Autodesk Inventor part; units mm, degrees
ref_plane "Work Plane1" through (0, 0, -15) normal (0, 0, 1) x (1, 0, 0)
ref_plane "YZ Plane" through (0, 0, 0) normal (1, 0, 0) x (0, 1, 0)
ref_plane "XZ Plane" through (0, 0, 0) normal (0, 1, 0) x (-1, 0, 0)
sketch "Sketch1" plane through (0, 0, 0) normal (0, 0, 1) x (1, 0, 0)
  line L0 (0, 0) -> (25, 0)
  line L1 (25, 0) -> (25, 40)
  line L2 (25, 40) -> (0, 40)
  line L3 (0, 40) -> (0, 0)
  dimension "d1" = 25
  dimension "d2" = 40
  dimension "d3" = 25
extrude "Extrusion1" add sketch "Sketch1" against normal blind 30
sketch "Sketch2" plane through (25, 0, 0) normal (1, 0, 0) x (0, 0, -1)
  line L0 (0, 0) -> (30, 0)
  circle A0 centre (15, 6.56) radius 2.46
extrude "Extrusion2" cut sketch "Sketch2" against normal blind 30
sketch "Sketch3" plane through (0, 0, 0) normal (-1, 0, 0) x (0, 0, 1)
  line L0 (0, 0) -> (-30, 0)
  line L1 (-25.05, 0) -> (-4.95, 0)
  line L2 (-4.95, 0) -> (-4.95, 33.12)
  line L3 (-4.95, 33.12) -> (-25.05, 33.12)
  line L4 (-25.05, 33.12) -> (-25.05, 0)
  dimension "d11" = 20.1
extrude "Extrusion3" cut sketch "Sketch3" against normal blind 20
sketch "Sketch4" plane through (0, 0, 0) normal (0, -1, 0) x (1, 0, 0)
  line L0 (20, -4.95) -> (20, -25.05)
  line L1 (20, -15) -> (25, -15)
  line L2 (25, 0) -> (25, -30)
  line L3 (20, -8.025) -> (25, -8.025)
  line L4 (25, -8.025) -> (25, -21.975)
  line L5 (25, -21.975) -> (20, -21.975)
  line L6 (20, -21.975) -> (20, -8.025)
  line L7 (20, -8.025) -> (25, -21.975) construction
  line L8 (25, -8.025) -> (20, -21.975) construction
  line L9 (25, -12.54) -> (25, -17.46)
  point P0 (0, 0)
  point P1 (22.5, -15)
  dimension "d14" = 13.95
extrude "Extrusion4" add sketch "Sketch4" along normal blind 15
sketch "Sketch5" plane through (20, 0, 0) normal (-1, 0, 0) x (0, 0, 1)
  circle A0 centre (-15, 6.56) radius 2.46
  circle A1 centre (-15, 6.56) radius 4.7025
  circle A2 centre (-15, 6.56) radius 2.46
  circle A3 centre (-15, 6.56) radius 2.46
  point P0 (0, 0)
  dimension "d17" = 9.405
extrude "Extrusion5" cut sketch "Sketch5" against normal blind 2.1
sketch "Sketch6" plane through (25, 0, 0) normal (1, 0, 0) x (0, 0, -1)
  circle A0 centre (15, 6.56) radius 4.7025
  line L0 (15, 6.56) -> (15, 23.56)
  circle A1 centre (15, 23.56) radius 2.46
  point P0 (0, 0)
  dimension "d20" = 17
  dimension "d21" = 4.92
extrude "Extrusion6" cut sketch "Sketch6" against normal blind 10 contours A1
sketch "Sketch7" plane through (20, 0, 0) normal (-1, 0, 0) x (0, 0, 1)
  circle A0 centre (-15, 23.56) radius 2.46
  circle A1 centre (-15, 23.56) radius 4.7025
  point P0 (0, 0)
  dimension "d24" = 9.405
extrude "Extrusion7" cut sketch "Sketch7" against normal blind 2.1
sketch "Sketch9" plane through (25, 0, 0) normal (1, 0, 0) x (0, 0, -1)
  circle A0 centre (15, 6.56) radius 2.46
  circle A1 centre (15, 6.56) radius 2.46
  circle A2 centre (15, 23.56) radius 2.46
  circle A3 centre (15, 23.56) radius 2.46
  line L0 (30, 40) -> (30, 0)
  line L1 (30, 0) -> (30, 40)
  line L2 (30, 40) -> (0, 40)
  line L3 (0, 40) -> (0, 0)
  line L4 (0, 0) -> (8.025, 0)
  line L5 (21.975, 0) -> (21.975, -15)
  line L6 (21.975, -15) -> (8.025, -15)
  line L7 (8.025, -15) -> (8.025, 0)
  line L8 (0, 0) -> (8.025, 0)
  line L9 (21.975, 0) -> (30, 0)
extrude "Extrusion8" add sketch "Sketch9" along normal blind 5
sketch "Sketch10" plane through (0, 40, 0) normal (0, 1, 0) x (1, 0, 0)
  line L0 (0, 30) -> (30, 30)
  line L1 (30, 0) -> (0, 0)
  line L2 (0, 30) -> (30, 30)
  line L3 (30, 30) -> (30, 0)
  line L4 (30, 0) -> (0, 0)
  line L5 (0, 0) -> (0, 30)
extrude "Extrusion9" add sketch "Sketch10" along normal blind 30
sketch "Sketch12" plane through (30, 0, 0) normal (1, 0, 0) x (0, 0, -1)
  circle A0 centre (15, 6.56) radius 2.46
  line L0 (15, 6.56) -> (15, 15.06)
  circle A1 centre (15, 15.06) radius 2.525
  point P0 (0, 0)
  dimension "d31" = 8.5
  dimension "d33" = 5.05
extrude "Extrusion10" cut sketch "Sketch12" against normal blind 30 contours A1
sketch "Sketch14" plane through (0, 0, 0) normal (0, 0, 1) x (1, 0, 0)
  line L0 (30, 70) -> (0, 70)
  line L1 (0, 70) -> (0, 85)
  line L2 (-15, 100) -> (-23, 100)
  line L3 (30, 0) -> (30, 70)
  line L4 (30, 118) -> (30, 70)
  arc A0 (0, 85) -> (-15, 100) centre (-15, 85) ccw
  line L5 (30, 105) -> (30, 100)
  line L6 (-18, 134) -> (-23, 136)
  line L7 (-18, 102) -> (-23, 100)
  line L8 (-18, 102) -> (-13, 118)
  line L9 (-13, 118) -> (-18, 134)
  line L10 (15, 136) -> (30, 118)
  line L11 (-23, 136) -> (15, 136)
  point P0 (0, 0)
  point P1 (0, 100)
  dimension "d47" = 30
  dimension "d54" = 15
extrude "Extrusion12" add sketch "Sketch14" against normal blind 30
sketch "Sketch15" plane through (0, 0, -25.05) normal (-1, 0, 0) x (0, 0, 1)
  line L0 (0, 33.12) -> (20.1, 33.12)
  line L1 (20.1, 33.12) -> (20.1, 0)
  line L2 (0, 33.12) -> (20.1, 33.12)
  line L3 (20.1, 33.12) -> (20.1, 31.1)
  line L4 (20.1, 31.1) -> (0, 31.1)
  line L5 (0, 31.1) -> (0, 33.12)
  point P0 (25.05, 0)
  dimension "d57" = 2.02
extrude "Extrusion13" add sketch "Sketch15" against normal blind 20
sketch "Sketch22" plane through (0, 0, 0) normal (0, 0, 1) x (1, 0, 0)
  line L0 (-15, 100) -> (-23, 100)
  line L1 (-15, 100) -> (-23, 100)
  line L2 (-23, 100) -> (-18, 102)
  line L3 (-23, 100) -> (-18, 102)
  line L4 (-18, 102) -> (-13, 118)
  line L5 (-18, 102) -> (-13, 118)
  line L6 (-13, 118) -> (-18, 134)
  line L7 (-13, 118) -> (-18, 134)
  line L8 (-18, 134) -> (-23, 136)
  line L9 (-18, 134) -> (-23, 136)
  line L10 (-23, 136) -> (15, 136)
  line L11 (-23, 136) -> (15, 136)
  line L12 (15, 136) -> (30, 118)
  line L13 (15, 136) -> (30, 118)
  line L14 (30, 118) -> (30, 78)
  line L15 (30, 0) -> (30, 118)
  line L16 (30, 78) -> (0, 78)
  arc A0 (0, 85) -> (-15, 100) centre (-15, 85) ccw
  line L17 (0, 78) -> (0, 85)
  arc A1 (0, 85) -> (-15, 100) centre (-15, 85) ccw
  point P0 (0, 0)
  dimension "d82" = 40
extrude "Extrusion14" add sketch "Sketch22" along normal blind 15
ref_plane "Work Plane1" through (0, 0, -15) normal (0, 0, 1) x (1, 0, 0)
mirror "Mirror1" about plane through (0, 0, -15) normal (0, 0, 1) of "Extrusion14"
properties part number "rec_a_32mm_x_60mm"
Can you work these out from the model? Positions are in its coordinate system, mm. A direction names the side the tool comes from. Coordinates: 2 decimals unless noted, no trailing zeros. Order: outer loops, then holes, each group sorted by start corner. A loop starts at its lowest first (then second) coordinate and runs counter-clockwise, first axis right, second up. Notation, with made-up numbers: (71.25, 35.5) - (112.25, 35.5) arc R20 ccw to (112.25, 58.5) - close; hole circle Ø8 at (76.25, 58). An arc over 180 degrees is marked (long way). Answer as a JSON object with one key per item and string values. Group by question number.
Q1. Imagine slicing it at B-B (y = 15.06). Please give me the cut outline in (x, z) (3 decimals), and give its area (4 significant figures).
Q2. We'd pull the mould along Z, two halves only. Please class faces 4 (the face through (25.07, 15.171, -12.477)), 5 (the face through (-15.465, 110.112, -14.58)), 6 (the face through (9, 107, 15)), 7 (the face through (25.995, 24.502, -17.272)): +Z half, -Z half, draft (parallel to the pull), parting line (faces both ways), or undercut.
Q3. Imagine slicing it at D-D (x = 10.5). Please give me the cut outline in (y, z).
Q4. Will these pins go through, and if not, where does the flat tip stop? P1, Ø16.5, axis at x = 13.5, z = 4, coming from the -Y side; P2, Ø6, axis at x = 0.5, z = -8.5, coming from the -Y side; P3, Ø15, axis at x = 17, y = 44.5, coming from the -Z side; P4, Ø6, axis at y = 15.06, z = -15, coming from the +X side.
Q5. On a 3-axis mill with a long thin cutter (end or side, diameter ignored), from which of +Z, -Z, +X, -X, +Y, -Y can I reach the whole of each face in a straight line? I mean faces 1 (the face through (15, 78, 7)), 2 (the face through (-19, 100, -15)), 3 (the face through (10, 15, -4.95)). Say none if no direction works.
Q6. Imagine slicing it at A-A (z = -15). Give the number of separate pieces and of enclosed holes in the cut face, and give its area (3 significant figures).
Q7. I need wall thicknesses on line 1 (Z direction, x = 23.5, y = 15.06) (3 decimals); line 2 (Y direction, x = 27.75, z = -15) (3 decimals); line 3 (Y direction, x = 28, z = -15) (3 decimals). Which ranges of each line are inside material? Lowest first, please. Write a range as from..to.
Q8. Imagine slicing it at C-C (z = -27). Please give me the cut outline in (x, y).
Determined:
{
 "1": {"outline": "(0, -30) - (30, -30) - (30, -17.525) - (20, -17.525) - (20, -25.05) - (0, -25.05) - close; (0, -4.95) - (20, -4.95) - (20, -12.475) - (30, -12.475) - (30, 0) - (0, 0) - close", "area": "447.5 mm2"},
 "2": {"face 4": "undercut", "face 5": "draft", "face 6": "+Z half", "face 7": "undercut"},
 "3": {"outline": "(0, -30) - (78, -30) - (78, -45) - (136, -45) - (136, 15) - (78, 15) - (78, 0) - (0, 0) - (0, -4.95) - (31.1, -4.95) - (31.1, -25.05) - (0, -25.05) - close"},
 "4": {"P1": "stops at y = 0", "P2": "stops at y = 31.1", "P3": "stops at z = -30", "P4": "stops at x = 30"},
 "5": {"face 1": "+Z, +X, -X, -Y", "face 2": "+Z, -Z, -X, -Y", "face 3": "-X, -Y"},
 "6": {"separate pieces": "4", "enclosed holes": "0", "area": "3,930 mm2"},
 "7": {"line 1": "z = -30..-17.525, -12.475..0", "line 2": "y = -15..4.1, 9.02..12.535, 17.585..21.1, 26.02..120.7", "line 3": "y = -15..4.1, 9.02..12.535, 17.585..21.1, 26.02..120.4"},
 "8": {"outline": "(-23, 100) - (-15, 100) arc R15 cw to (0, 85) - (0, 0) - (30, 0) - (30, 118) - (15, 136) - (-23, 136) - (-18, 134) - (-13, 118) - (-18, 102) - close"}
}
